The model under review builds one solid part; all positions refer to its coordinate system, in mm. A direction names the side the tool comes from. Round coordinates to 2 decimals unless told otherwise and drop trailing zeros. Order: outer loops, then holes, each group sorted by start corner. A loop starts at its lowest first (then second) coordinate and runs counter-clockwise, first axis right, second up. Notation, with made-up numbers: (40.25, 32) -> (50.25, 32) arc R15 cw to (50.25, 43) -> close; hole circle Ø11 at (52.5, 77). An arc over 180 degrees is marked (long way). Use a Markdown table: item, result. Add a question column.
```python
from build123d import *

# Parameters (mm, degrees)
SKETCH1_W           = 15
SKETCH1_H           = 15
BOSS_EXTRUDE1_DEPTH = 0.8
BOSS_EXTRUDE2_DEPTH = 1
SKETCH3_R           = 0.75
CUT_EXTRUDE2_DEPTH  = 9.5
SKETCH6_R           = 0.75
CUT_EXTRUDE3_DEPTH  = 70


with BuildPart() as part:
    # Sketch1 → Boss-Extrude1 (new body)
    with BuildSketch(Plane(origin=(0, 0, 0), x_dir=(1, 0, 0), z_dir=(0, 1, 0))):
        Rectangle(SKETCH1_W, SKETCH1_H)
    extrude(amount=BOSS_EXTRUDE1_DEPTH)

    # Sketch2 → Boss-Extrude2 (add, symmetric)
    with BuildSketch(Plane.XY):
        with BuildLine():
            Line((-7.5, 0.8), (6.263352991, 20.848942976))
            ThreePointArc((6.263352991, 20.848942976), (8.00009228, 21.414180933), (8.995415357, 19.8828125))
            Line((8.995415357, 19.8828125), (7.5, 0.8))
            Line((7.5, 0.8), (-7.5, 0.8))
        make_face()
    extrude(amount=BOSS_EXTRUDE2_DEPTH, both=True)

    # Sketch3 → Cut-Extrude2 (cut, through all)
    with BuildSketch(Plane(origin=(0, 0, -1), x_dir=(-1, 0, 0), z_dir=(0, 0, -1))):
        with Locations((-7.5, 20)):
            Circle(SKETCH3_R)
    extrude(amount=-CUT_EXTRUDE2_DEPTH, mode=Mode.SUBTRACT)

    # Sketch6 → Cut-Extrude3 (cut)
    with BuildSketch(Plane.XY.offset(1)):
        with Locations((6.803358906, 14.3)):
            Circle(SKETCH6_R)
        with Locations((6.295860941, 8.8)):
            Circle(SKETCH6_R)
        Polygon((-2.039936244, 6.986718852), (-5.293464788, 2.247335339), (4.863877808, 2.247335339), align=None)
        Polygon((-1.47397426, 7.811150191), (4.556357867, 3.671401287), (2.597993052, 13.742745529), align=None)
    extrude(amount=-CUT_EXTRUDE3_DEPTH, mode=Mode.SUBTRACT)


solid = part.part
```
Q1. Add section B-B, the plane x = -3.75. Give the boundary of the cut face in (y, z).
Q2. Add section A-A, the plane y = 11.5. Give the boundary of the cut face in (x, z).
Q3. For pin 1 (0.9 mm diameter, centred on x = 6.3, y = 8.8, fed in from +Z); pin 2 (2 mm diameter, centred on x = -2, z = -4.5, fed in from +Y); pin 3 (2 mm diameter, centred on x = 7, y = 17, fed in from -Z); pin 4 (1.5 mm diameter, centred on y = 9, z = -1, fed in from -X), all flat-tipped, find the tip position at first contact; note any pin that passes through.
Q4. Draft analysis for pull direction Y (two halves, no side actions). For faces 6 (the face through (1.46, 4.584, 0.014)), 7 (the face through (0, 0.8, 4)), 8 (the face through (0, 0, 0)), state which applies: released by +Y, released by -Y, zero draft, split by the parting line, or undercut.
Q5. For faces 1 (the face through (-0.715, 10.684, 0.014)), 2 (the face through (5, 9, 1)), 3 (the face through (5, 9, -1)), 4 (the face through (8.258, 10.475, 0.014)), 5 (the face through (0, 2.247, 0)), list the 3-axis set-ups (+Z, -Z, +X, -X, +Y, -Y) from which the entire face can be reached by the end or side of a thin tool; tool diameter is ignored.
Q6. Add section C-C, the plane y = 8.8. Give the boundary of the cut face in (x, z).
Q7. To check wall thickness, follow line 1 along Y through (x, z) = (-0.75, 0.25); line 2 along Y through (x, z) = (1.5, 3.75); line 3 along Y through (x, z) = (-3.25, -0.25). State the ranges of each line that lie inside material, in increasing order.
Q8. Add section D-D, the plane x = 0. Give the boundary of the cut face in (y, z).
Return value:
| question | item | result |
|---|---|---|
| 1 | outline | (0, -7.5) -> (0.8, -7.5) -> (0.8, -1) -> (2.25, -1) -> (2.25, 1) -> (0.8, 1) -> (0.8, 7.5) -> (0, 7.5) -> close; (4.5, -1) -> (6.26, -1) -> (6.26, 1) -> (4.5, 1) -> close |
| 2 | outline | (-0.15, -1) -> (1.06, -1) -> (1.06, 1) -> (-0.15, 1) -> close; (3.03, -1) -> (8.34, -1) -> (8.34, 1) -> (3.03, 1) -> close |
| 3 | pin 1 | through |
| 3 | pin 2 | y = 0.8 |
| 3 | pin 3 | z = -1 |
| 3 | pin 4 | x = -2.39 |
| 4 | face 6 | undercut |
| 4 | face 7 | released by +Y |
| 4 | face 8 | released by -Y |
| 5 | face 1 | +Z, -Z, -X, +Y |
| 5 | face 2 | +Z, +X, -X, +Y |
| 5 | face 3 | -Z, +X, -X, +Y |
| 5 | face 4 | +Z, -Z, +X, -Y |
| 5 | face 5 | +Z, -Z |
| 6 | outline | (-2.01, -1) -> (-0.8, -1) -> (-0.8, 1) -> (-2.01, 1) -> close; (3.56, -1) -> (5.55, -1) -> (5.55, 1) -> (3.56, 1) -> close; (7.05, -1) -> (8.13, -1) -> (8.13, 1) -> (7.05, 1) -> close |
| 7 | line 1 | 0 to 2.25, 6.1 to 7.31, 8.87 to 10.63 |
| 7 | line 2 | 0 to 0.8 |
| 7 | line 3 | 0 to 2.25, 5.22 to 6.99 |
| 8 | outline | (0, -7.5) -> (0.8, -7.5) -> (0.8, -1) -> (2.25, -1) -> (2.25, 1) -> (0.8, 1) -> (0.8, 7.5) -> (0, 7.5) -> close; (5.59, -1) -> (6.8, -1) -> (6.8, 1) -> (5.59, 1) -> close; (9.96, -1) -> (11.73, -1) -> (11.73, 1) -> (9.96, 1) -> close |
